Verification items for the finished model (mm, model axes). A direction names the side the tool comes from. Round coordinates to 2 decimals unless told otherwise and drop trailing zeros. Write each loop counter-clockwise with the first axis right and the second up, starting at its lowest first coordinate (ties: lowest second). Pieces come first, ordered by that corner, then holes. Notation, with made-up numbers: M 33,-19.75 L 40,-19.75 A23 cw 40,14.25 Z; hole C 47,7.25 d8. An arc over 180 degrees is marked long. One line per item, written item: value. Start each with the question number.
Autodesk Inventor part; units mm, degrees
ref_plane "YZ Plane" through (0, 0, 0) normal (1, 0, 0) x (0, 1, 0)
ref_plane "XZ Plane" through (0, 0, 0) normal (0, 1, 0) x (-1, 0, 0)
ref_plane "XY Plane" through (0, 0, 0) normal (0, 0, 1) x (1, 0, 0)
sketch "Sketch1" plane through (0, 0, 0) normal (0, 1, 0) x (-1, 0, 0)
  line L0 (25.1574, 62.1971) -> (0, 62.1971)
  line L1 (0, 62.1971) -> (0, 0)
  line L2 (0, 0) -> (181.61, 0)
  line L3 (181.61, 0) -> (181.61, 62.1971)
  line L4 (181.61, 62.1971) -> (27.6626, 62.1971)
  line L5 (4.96, 54.5289) -> (44.2742, 54.5289)
  line L6 (44.2742, 54.5289) -> (50.5671, 48.2322)
  line L7 (50.5671, 48.2322) -> (50.5671, 31.808)
  line L8 (50.5671, 31.808) -> (44.2742, 25.5113)
  line L9 (44.2742, 25.5113) -> (4.96, 25.5113)
  ellipse E0 centre (69.3942, 20.866) end of major axis (69.3942, 10.8599) minor radius 10
  ellipse E1 centre (69.3942, 50.8843) end of major axis (69.3942, 40.8782) minor radius 10
  ellipse E2 centre (109.3942, 20.866) end of major axis (109.3942, 10.8599) minor radius 10
  ellipse E3 centre (109.3942, 50.8843) end of major axis (109.3942, 40.8782) minor radius 10
  ellipse E4 centre (149.3942, 50.8843) end of major axis (149.3942, 40.8782) minor radius 10
  ellipse E5 centre (149.3942, 20.866) end of major axis (149.3942, 10.8599) minor radius 10
  ellipse E6 centre (26.41, 60.0323) end of major axis (26.41, 57.5308) minor radius 2.5 (25.1574, 62.1971) -> (27.6626, 62.1971) ccw
  ellipse E7 centre (4.96, 51.5271) end of major axis (4.96, 48.5253) minor radius 3 (4.96, 54.5289) -> (1.96, 51.5271) ccw
  ellipse E8 centre (4.96, 28.5131) end of major axis (4.96, 25.5113) minor radius 3 (1.96, 28.5131) -> (4.96, 25.5113) ccw
  line L10 (1.96, 28.5131) -> (1.96, 51.5271)
  ellipse E9 centre (26.41, 20.0079) end of major axis (26.41, 17.7565) minor radius 2.25
  point P0 (27.6626, 62.1971)
extrude "Extrusion1" add sketch "Sketch1" along normal blind 3
properties part number "EboxSide"
1) Mould release check, pull along Y, two halves, no side actions. Record for faces 1 (the flat face through (-90, 3, 25)), 2 (the flat face through (-50.567, 1, 40)), 3 (the flat face through (-90, 0, 25)): pulls with the +Y half, pulls with the -Y half, needs draft (parallel to the pull), parting line crosses it, or undercut.
2) Cross-section at A-A (x = -10.5). Record the boundary of the cut face in (y, z), then the cut area to 3 significant figures.
3) Gauge pin test, flat end, axial feed: pin 1 Ø12 at (x, z) = (-113.5, 11) entering from -Y. Record the tip position at first contact, or that the pin passes through.
4) Thickness scan on line 1 (X direction, y = 2.05, z = 17); line 2 (Z direction, x = -105.5, y = 0.6); line 3 (Z direction, x = -29.5, y = 0.6). Record the ranges inside material, lowest first.
5) Cross-section at B-B (z = 35.5). Record the boundary of the cut face in (x, y), then the cut area to 3 significant figures.
6) Cross-section at C-C (y = 1.45). State how many separate pieces and enclosed holes the cut face has, then the cut area to 3 significant figures.
7) Access from +Z, -Z, +X, -X, +Y, -Y to the whole of each face (thin tool, end or side, straight path). Record for faces 4 (the flat face through (0, 1, 32)), 5 (the flat face through (-1.96, 1, 40)).
Results below:
1. face 1: pulls with the +Y half
1. face 2: needs draft
1. face 3: pulls with the -Y half
2. outline: M 0,0 L 3,0 L 3,25.51 L 0,25.51 Z; M 0,54.53 L 3,54.53 L 3,62.2 L 0,62.2 Z
2. area: 99.5 mm²
3. pin 1: stops at y = 0
4. line 1: x = -181.61 to -158.62, -140.17 to -118.62, -100.17 to -78.62, -60.17 to 0
4. line 2: z = 0 to 11.65, 30.08 to 41.67, 60.1 to 62.2
4. line 3: z = 0 to 25.51, 54.53 to 62.2
5. outline: M -181.61,0 L -50.57,0 L -50.57,3 L -181.61,3 Z; M -1.96,0 L 0,0 L 0,3 L -1.96,3 Z
5. area: 399 mm²
6. separate pieces: 1
6. enclosed holes: 8
6. area: 8,010 mm²
7. face 4: +Z, -Z, +X, +Y, -Y
7. face 5: +Y, -Y
